```python
from build123d import *

# Parameters (mm, degrees)
SKETCH_1_R          = 1.15
EXTRUDE_1_DEPTH     = 3
SKETCH_2_W          = 13.26
SKETCH_2_H          = 4.63
SKETCH_2_H_2        = 4.947868295
EXTRUDE_2_DEPTH     = 12.36
SKETCH_3_R          = 1
CUT_EXTRUDE_1_DEPTH = 100


with BuildPart() as part:
    # 草图1 → 凸台-拉伸1 (new body)
    with BuildSketch(Plane.XY):
        Polygon((-32.300556088, -10.432591376), (-32.300556088, 17.427408624), (-19.040556088, 17.427408624), (-19.040556088, -10.432591376), (19.033443912, -10.432591376), (19.033443912, 17.427408624), (32.293443912, 17.427408624), (32.293443912, -10.432591376), (40.493443912, -10.432591376), (40.493443912, -17.112591376), (-40.500556088, -17.112591376), (-40.500556088, -10.432591376), align=None)
        with Locations((-35.300556088, -13.772591376)):
            Circle(SKETCH_1_R, mode=Mode.SUBTRACT)
        with Locations((-24.300556088, -13.772591376)):
            Circle(SKETCH_1_R, mode=Mode.SUBTRACT)
        with Locations((24.299443912, -13.772591376)):
            Circle(SKETCH_1_R, mode=Mode.SUBTRACT)
        with Locations((35.299443912, -13.772591376)):
            Circle(SKETCH_1_R, mode=Mode.SUBTRACT)
    extrude(amount=EXTRUDE_1_DEPTH)

    # 草图2 → 凸台-拉伸2 (add)
    with BuildSketch(Plane.XY.offset(3)):
        with Locations((-25.670556088, 15.112408624)):
            Rectangle(SKETCH_2_W, SKETCH_2_H)
        with Locations((25.663443912, 14.953474477)):
            Rectangle(SKETCH_2_W, SKETCH_2_H_2)
    extrude(amount=EXTRUDE_2_DEPTH)

    # 草图3 → 切除-拉伸1 (cut)
    with BuildSketch(Plane.ZY.offset(32.300556088)):
        with Locations((9.36, 15.427408624)):
            Circle(SKETCH_3_R)
    extrude(amount=-CUT_EXTRUDE_1_DEPTH, mode=Mode.SUBTRACT)


solid = part.part
```
Input: part model. Units: mm. Frame: model coordinates. A direction names the side the tool comes from. Round coordinates to 2 decimals unless told otherwise and drop trailing zeros. Write each loop counter-clockwise with the first axis right and the second up, starting at its lowest first coordinate (ties: lowest second). Pieces come first, ordered by that corner, then holes. Notation, with made-up numbers: (10.25, -13) - (15.25, -13) arc R14 ccw to (15.25, 13) - close; hole circle Ø9 at (-15.75, 41.25). An arc over 180 degrees is marked (long way). Write item = value, one per line.
(1) Section query A-A on y = -1.5. Output: boundary loops of the cut face in (x, z).
Geometry check:
outline = (-32.3, 0) - (-19.04, 0) - (-19.04, 3) - (-32.3, 3) - close; (19.03, 0) - (32.29, 0) - (32.29, 3) - (19.03, 3) - close
(2) Contact query for flat-ended pins moving along their axis: pin 1 Ø1.5 at (x, z) = (8, 1.5) entering from +Y; pin 2 Ø7.5 at (y, z) = (-1.5, 6.5) entering from -X; pin 3 Ø5 at (x, y) = (28, -5) entering from +Z. Output: stop coordinate, or through.
Geometry check:
pin_1 = -10.43
pin_2 = -32.3
pin_3 = 3
(3) Section query D-D on x = 26.5. Output: boundary loops of the cut face in (y, z), then the cut area to 3 significant figures.
Geometry check:
outline = (-17.11, 0) - (17.43, 0) - (17.43, 15.36) - (12.48, 15.36) - (12.48, 3) - (-17.11, 3) - close; hole circle Ø2 at (15.43, 9.36)
area = 162 mm^2
(4) Pull-direction query (X, two-part tool) for faces 6 (the cylindrical face through (-25.76, 14.45, 9.14)), 7 (the flat face through (32.293, 7, 2)), 8 (the cylindrical face through (25.396, -13.427, 1.479)); classes: +X half, -X half, draft (parallel to the pull), parting line (faces both ways), or undercut.
Geometry check:
face_6 = draft
face_7 = +X half
face_8 = undercut
(5) Access query for faces 1 (the flat face through (26, 12.48, 9)), 2 (the flat face through (-26, 12.797, 9)), 3 (the flat face through (-36, -10.433, 1)), 4 (the flat face through (-19.041, 6.5, 2.5)), 5 (the flat face through (36, -10.433, 1)). Directions: +Z, -Z, +X, -X, +Y, -Y. A direction counts if a zero-diameter tool reaches every point of the face in a straight line with its end or side. Return the directions, or none.
Geometry check:
face_1 = +Z, +X, -X, -Y
face_2 = +Z, -X, -Y
face_3 = +Z, -Z, -X, +Y
face_4 = +Z, -Z, +Y
face_5 = +Z, -Z, +X, +Y
(6) Section query B-B on z = 13.75. Output: boundary loops of the cut face in (x, y), then the cut area to 3 significant figures.
Geometry check:
outline = (-32.3, 12.8) - (-19.04, 12.8) - (-19.04, 17.43) - (-32.3, 17.43) - close; (19.03, 12.48) - (32.29, 12.48) - (32.29, 17.43) - (19.03, 17.43) - close
area = 127 mm^2
(7) Section query C-C on z = 9.36. Output: boundary loops of the cut face in (x, y).
Geometry check:
outline = (-32.3, 12.8) - (-19.04, 12.8) - (-19.04, 14.43) - (-32.3, 14.43) - close; (-32.3, 16.43) - (-19.04, 16.43) - (-19.04, 17.43) - (-32.3, 17.43) - close; (19.03, 12.48) - (32.29, 12.48) - (32.29, 14.43) - (19.03, 14.43) - close; (19.03, 16.43) - (32.29, 16.43) - (32.29, 17.43) - (19.03, 17.43) - close
(8) Material intervals for probe 1 along Y at (x, z) = (22, 9.36); probe 2 along Y at (x, z) = (-30, 14.25); probe 3 along Y at (x, z) = (-20.5, 9.5), sorted ascending.
Geometry check:
probe_1 = 12.48 to 14.43, 16.43 to 17.43
probe_2 = 12.8 to 17.43
probe_3 = 12.8 to 14.44, 16.42 to 17.43
